Build history of the part. All positions in model axes, mm. A direction names the side the tool comes from. Coordinates: 2 decimals unless noted, no trailing zeros. Loops run counter-clockwise (first coordinate to the right, second up) from the corner with the lowest first, then second, coordinate; pieces in that order, holes last.
Item 1: Drill centre lines: line 1 along X through (y, z) = (42, -12); line 2 along X through (y, z) = (41.7, -29.5); line 3 along X through (y, z) = (44, -29). Where is each one in solid material? Low to high.
Item 2: Flat gauge pins, fed straight in: pin 1 (0.9 mm diameter, centred on y = 41.5, z = -20.5, fed in from +X); pin 2 (2.5 mm diameter, centred on y = 42, z = 7, fed in from +X); pin 3 (10 mm diameter, centred on y = 41.5, z = -48, fed in from +X). Where does each tip first touch, or does it go through?
Item 3: Cut at B-B (y = 22). List the corners of the cut face in (x, z).
Item 4: 3-axis set-ups, long thin cutter, end or side, ignore diameter. For faces 4 (the face through (49.67, 14.65, 50.04)), 5 (the face through (-24, 50.8, -5)), 6 (the face through (-64.01, 14.65, 29.56)), 7 (the face through (-49.67, 14.65, 50.04)): which of +Z, -Z, +X, -X, +Y, -Y reach the whole face in a straight line?
Item 5: Cut at C-C (y = 34). List the corners of the cut face in (x, z).
Item 6: Mould opens along X. For faces 1 (the face through (-69.483, 14.652, -11.987)), 2 (the face through (-6, 0, 62)), 3 (the face through (-44.835, 42.689, 48.895)) say: released by +X, released by -X, zero draft, split by the parting line, or undercut.
from build123d import *

# Parameters (mm, degrees)
CUT_EXTRUDE1_DEPTH         = 40.2
SKETCH5_R                  = 13.1
CUT_EXTRUDE2_DEPTH         = 10.6
BOSS_EXTRUDE1_START        = 3.175
SKETCH5_3_R                = 24
SKETCH5_3_R_2              = 13.1
BOSS_EXTRUDE1_DEPTH        = 3.175
SKETCH6_W                  = 25
SKETCH6_H                  = 28.783830664
CUT_EXTRUDE3_DEPTH         = 46.8
CIRPATTERN1_COUNT          = 3
CIRPATTERN1_ANGLE          = 110
CIRPATTERN2_COUNT          = 3
CIRPATTERN2_ANGLE          = 110
SKETCH7_W                  = 26.05355805
SKETCH7_H                  = 46.414815382
CUT_EXTRUDE4_DEPTH         = 2.95
M2_5_CLEARANCE_HOLE1_D     = 2.9
M2_5_CLEARANCE_HOLE1_DEPTH = 6
M2_5_CLEARANCE_HOLE1_TIP   = 0.871247898
SKETCH11_R                 = 57.15
SKETCH11_R_2               = 31.75
CUT_EXTRUDE5_DEPTH         = 2.54


with BuildPart() as part:
    # Sketch3 → Revolve1 (revolve)
    with BuildSketch(Plane.XY, mode=Mode.PRIVATE) as revolve1_sk:
        Polygon((60.96, 0), (81.28, 0), (63.5, 50.8), (0, 50.8), (0, 0), align=None)
    revolve(revolve1_sk.sketch.rotate(Axis((0, 0, 0), (0, 1, 0)), 90), axis=Axis((0, 0, 0), (0, 1, 0)))

    # Sketch4 → Cut-Extrude1 (cut)
    with BuildSketch(Plane(origin=(0, 0, 0), x_dir=(-1, 0, 0), z_dir=(0, -1, 0))):
        with BuildLine():
            Line((-44.999992712, 39.078902952), (-44.999992712, 81.540670454))
            Line((-44.999992712, 81.540670454), (44.999992712, 81.540670454))
            Line((44.999992712, 81.540670454), (44.999992712, 39.078902952))
            ThreePointArc((44.999992712, 39.078902952), (0, -59.6), (-44.999992712, 39.078902952))
        make_face()
    extrude(amount=-CUT_EXTRUDE1_DEPTH, mode=Mode.SUBTRACT)

    # Sketch5 → Cut-Extrude2 (cut)
    with BuildSketch(Plane(origin=(0, 50.8, 0), x_dir=(1, 0, 0), z_dir=(0, 1, 0))):
        with Locations(Location((0, 0, 0), (0, 0, 270))):
            Circle(SKETCH5_R)
    extrude(amount=-CUT_EXTRUDE2_DEPTH, mode=Mode.SUBTRACT)

    # Sketch5<3> → Boss-Extrude1 (add)
    with BuildSketch(Plane(origin=(0, 50.8, 0), x_dir=(1, 0, 0), z_dir=(0, 1, 0)).offset(BOSS_EXTRUDE1_START)):
        with Locations(Location((0, 0, 0), (0, 0, 270))):
            Circle(SKETCH5_3_R)
        with Locations(Location((0, 0, 0), (0, 0, 270))):
            Circle(SKETCH5_3_R_2, mode=Mode.SUBTRACT)
    extrude(amount=-BOSS_EXTRUDE1_DEPTH)

    # Sketch6 → Cut-Extrude3 (cut)
    with BuildSketch(Plane(origin=(0, 50.8, 0), x_dir=(1, 0, 0), z_dir=(0, 1, 0))):
        with Locations((0, -80)):
            Rectangle(SKETCH6_W, SKETCH6_H)
    cut_extrude3 = extrude(amount=-CUT_EXTRUDE3_DEPTH, mode=Mode.SUBTRACT)

    # CirPattern1: Cut-Extrude3 ×3 about axis
    cirpattern1_axis = Axis((0, 0, 0), (0, -1, 0))
    for i in range(1, CIRPATTERN1_COUNT):
        add(cut_extrude3.rotate(cirpattern1_axis, i * CIRPATTERN1_ANGLE / (CIRPATTERN1_COUNT - 1)), mode=Mode.SUBTRACT)

    # CirPattern2: Cut-Extrude3 ×3 about axis
    cirpattern2_axis = Axis((0, 0, 0), (0, 1, 0))
    for i in range(1, CIRPATTERN2_COUNT):
        add(cut_extrude3.rotate(cirpattern2_axis, i * CIRPATTERN2_ANGLE / (CIRPATTERN2_COUNT - 1)), mode=Mode.SUBTRACT)

    # Sketch7 → Cut-Extrude4 (cut)
    with BuildSketch(Plane.XZ.offset(-40.2)):
        with Locations((0, -4.57891024)):
            Rectangle(SKETCH7_W, SKETCH7_H)
    extrude(amount=-CUT_EXTRUDE4_DEPTH, mode=Mode.SUBTRACT)

    # M2.5 Clearance Hole1
    with Locations(Plane(origin=(0, 40.2, 0), x_dir=(-1, 0, 0), z_dir=(0, -1, 0))):
        with Locations((-15, -4.5), (15, -4.5), (15, 12.5), (-15, 12.5), (15, 29.5), (-15, 29.5), (-8.5, 35.8), (8.5, 35.8)):
            Hole(M2_5_CLEARANCE_HOLE1_D / 2, depth=M2_5_CLEARANCE_HOLE1_DEPTH)
            with Locations((0, 0, -(M2_5_CLEARANCE_HOLE1_DEPTH + M2_5_CLEARANCE_HOLE1_TIP / 2))):  # 118° drill point
                Cone(0, M2_5_CLEARANCE_HOLE1_D / 2, M2_5_CLEARANCE_HOLE1_TIP, mode=Mode.SUBTRACT)

    # Sketch11 → Cut-Extrude5 (cut)
    with BuildSketch(Plane(origin=(0, 50.8, 0), x_dir=(1, 0, 0), z_dir=(0, 1, 0))):
        with Locations(Location((0, 0, 0), (0, 0, 270))):
            Circle(SKETCH11_R)
        with Locations(Location((0, 0, 0), (0, 0, 270))):
            Circle(SKETCH11_R_2, mode=Mode.SUBTRACT)
    extrude(amount=-CUT_EXTRUDE5_DEPTH, mode=Mode.SUBTRACT)


solid = part.part
Filled sheet:
1. line 1: x = -65.45 to -16.36, -13.64 to -13.03, 13.03 to 13.64, 16.36 to 65.45
1. line 2: x = -59.08 to -16.45, -13.55 to 13.55, 16.45 to 59.08
1. line 3: x = -59.15 to -16.36, -13.64 to 13.64, 16.36 to 59.15
2. pin 1: stops at x = 62.52
2. pin 2: stops at x = 66.67
2. pin 3: stops at x = 51.64
3. outline: (-72.41, -13.05) - (-65.93, -10.69) - (-57.38, -34.19) - (-63.86, -36.55) arc R73.58 ccw to (-45, -58.22) - (-45, -39.08) arc R59.6 cw (long way) to (45, -39.08) - (45, -58.22) arc R73.58 ccw to (63.86, -36.55) - (57.38, -34.19) - (65.93, -10.69) - (72.41, -13.05) arc R73.58 ccw to (66.57, 31.35) - (60.91, 27.39) - (46.57, 47.87) - (52.23, 51.83) arc R73.58 ccw to (12.5, 72.51) - (12.5, 65.61) - (-12.5, 65.61) - (-12.5, 72.51) arc R73.58 ccw to (-52.23, 51.83) - (-46.57, 47.87) - (-60.91, 27.39) - (-66.57, 31.35) arc R73.58 ccw to start
4. face 4: +X, +Y
4. face 5: +Y
4. face 6: +Z, +Y
4. face 7: -X, +Y
5. outline: (-68.4, -11.59) - (-65.93, -10.69) - (-57.38, -34.19) - (-59.85, -35.09) arc R69.38 ccw to (-45, -52.81) - (-45, -39.08) arc R59.6 cw (long way) to (45, -39.08) - (45, -52.81) arc R69.38 ccw to (59.85, -35.09) - (57.38, -34.19) - (65.93, -10.69) - (68.4, -11.59) arc R69.38 ccw to (63.07, 28.9) - (60.91, 27.39) - (46.57, 47.87) - (48.73, 49.38) arc R69.38 ccw to (12.5, 68.24) - (12.5, 65.61) - (-12.5, 65.61) - (-12.5, 68.24) arc R69.38 ccw to (-48.73, 49.38) - (-46.57, 47.87) - (-60.91, 27.39) - (-63.07, 28.9) arc R69.38 ccw to start
6. face 1: undercut
6. face 2: zero draft
6. face 3: split by the parting line
